```python
from build123d import *

# Parameters (mm, degrees)
F0_W     = 20
F0_H     = 20
F1_DEPTH = 20
F3_W     = 20
F3_H     = 20
F3_R     = 2.6
F6_DEPTH = 1
F5_R     = 2.6
F4_R     = 2.6
F8_DEPTH = 2


with BuildPart() as f1:
    # F0 (on Front) → F1 (new body)
    with BuildSketch(Plane.XZ):
        with Locations((10, 10)):
            Rectangle(F0_W, F0_H)
    extrude(amount=F1_DEPTH)

    # F3 (on face) → F6 (cut)
    with BuildSketch(Plane(origin=(0, 0, 0), x_dir=(-1, 0, 0), z_dir=(0, 1, 0))):
        with Locations((-10, 10)):
            Rectangle(F3_W, F3_H)
        with Locations((-15, 5)):
            Circle(F3_R, mode=Mode.SUBTRACT)
        with Locations((-5, 5)):
            Circle(F3_R, mode=Mode.SUBTRACT)
        with Locations((-15, 15)):
            Circle(F3_R, mode=Mode.SUBTRACT)
        with Locations((-10, 10)):
            Circle(F3_R, mode=Mode.SUBTRACT)
        with Locations((-5, 15)):
            Circle(F3_R, mode=Mode.SUBTRACT)
        with Locations((-5, 15)):
            Circle(F3_R)
    extrude(amount=-F6_DEPTH, mode=Mode.SUBTRACT)

    # F5 (on face) + F4 (on face) → F8 (cut)
    with BuildSketch(Plane(origin=(0, 0, 0), x_dir=(-1, 0, 0), z_dir=(0, 1, 0))):
        with Locations((-15, 15)):
            Circle(F5_R)
        with Locations((-5, 15)):
            Circle(F5_R)
        with Locations((-10, 10)):
            Circle(F5_R)
        with Locations((-5, 5)):
            Circle(F5_R)
    with BuildSketch(Plane(origin=(0, 0, 0), x_dir=(-1, 0, 0), z_dir=(0, 1, 0))):
        with Locations((-15, 5)):
            Circle(F4_R)
    extrude(amount=-F8_DEPTH, mode=Mode.SUBTRACT)


solid = f1.part
```
For this review, take the finished solid that the model builds, in its own axes (mm). A direction names the side the tool comes from. Round coordinates to 2 decimals unless told otherwise and drop trailing zeros. Write each loop counter-clockwise with the first axis right and the second up, starting at its lowest first coordinate (ties: lowest second). Pieces come first, ordered by that corner, then holes. Notation, with made-up numbers: (7, 56.5) -> (22, 56.5) arc R24 cw to (22, 87.5) -> close; hole circle Ø8 at (33.5, -26). An arc over 180 degrees is marked (long way). One line per question, with ' | ' between items. Start each with the question number.
1) Machinability: for faces 1 (the flat face through (10, -20, 10)), 2 (the flat face through (5, -2, 15)), which of the approach directions +Z, -Z, +X, -X, +Y, -Y give a long, thin tool a straight path to every point of the face, cutting with its end or side? Answer none if there is none.
2) Add section B-B (z = 5). Write out the cut boundary in (x, y), and give its area (3 significant figures).
3) Add section A-A (x = 5). Write out the cut boundary in (y, z).
4) For pin 1 Ø4 at (x, z) = (5, 14.5) entering from +Y, flat-tipped, find the tip position at first contact; note if it passes through.
5) Wall thickness on line 1 along Z through (x, y) = (15, -1.5); line 2 along Y through (x, z) = (10.75, 10.25): over which ranges is each line inside the solid? List them lowest first.
Reported:
1) face 1: +Z, -Z, +X, -X, -Y | face 2: +Y
2) outline: (0, -20) -> (20, -20) -> (20, -1) -> (17.6, -1) -> (17.6, -2) -> (12.4, -2) -> (12.4, -1) -> (7.6, -1) -> (7.6, -2) -> (2.4, -2) -> (2.4, -1) -> (0, -1) -> close | area: 370 mm²
3) outline: (-20, 0) -> (-1, 0) -> (-1, 2.4) -> (-2, 2.4) -> (-2, 7.6) -> (-1, 7.6) -> (-1, 12.4) -> (-2, 12.4) -> (-2, 17.6) -> (-1, 17.6) -> (-1, 20) -> (-20, 20) -> close
4) pin 1: stops at y = -2
5) line 1: z = 0 to 2.4, 7.6 to 12.4, 17.6 to 20 | line 2: y = -20 to -2
